Source: CAD feature listing. Evaluate the final solid. Frame: model axes, mm. Give positions to 0.01 mm unless a question says otherwise; leave off trailing zeros. Write each loop counter-clockwise with the first axis right and the second up, starting at its lowest first coordinate (ties: lowest second). Pieces come first, ordered by that corner, then holes. Notation, with made-up numbers: M 42.25,3 L 70.25,3 A22 cw 70.25,36 Z; hole C 70.25,51.5 d10. An arc over 180 degrees is marked long. Answer as a JSON object with one key per item and string values. Group by question number.
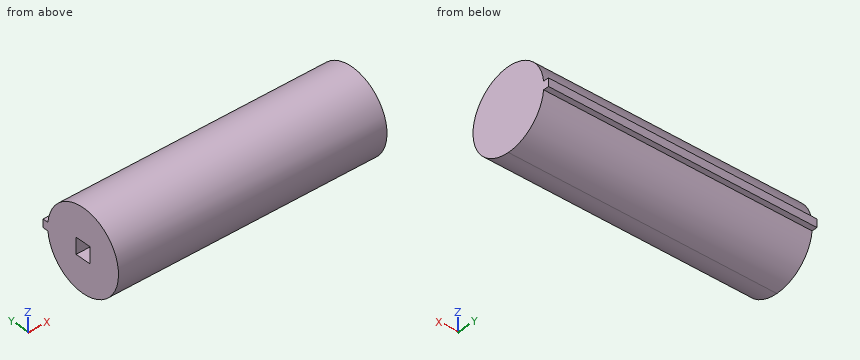
```python
from build123d import *

# Parameters (mm, degrees)
EXTRUDE_1_DEPTH     = 100
SKETCH_2_W          = 6
SKETCH_2_H          = 6
CUT_EXTRUDE_1_DEPTH = 15


with BuildPart() as part:
    # 草图1 → 凸台-拉伸1 (new body)
    with BuildSketch(Plane(origin=(0, 0, 0), x_dir=(0, 0, -1), z_dir=(1, 0, 0))):
        with BuildLine():
            Line((-1.5, 14.924811557), (-1.5, 0))
            Line((-1.5, 0), (1.5, 0))
            Line((1.5, 0), (1.5, 14.924811557))
            ThreePointArc((1.5, 14.924811557), (0, 15), (-1.5, 14.924811557))
        make_face()
        with BuildLine():
            Line((1.5, 0), (-1.5, 0))
            Line((-1.5, 0), (-1.5, 14.924811557))
            ThreePointArc((-1.5, 14.924811557), (-10.062305899, -11.124297731), (15, 0))
            ThreePointArc((15, 0), (11.124297731, 10.062305899), (1.5, 14.924811557))
            Line((1.5, 14.924811557), (1.5, 0))
        make_face()
        with BuildLine():
            Line((-1.5, 17), (-1.5, 14.924811557))
            ThreePointArc((-1.5, 14.924811557), (0, 15), (1.5, 14.924811557))
            Line((1.5, 14.924811557), (1.5, 17))
            Line((1.5, 17), (-1.5, 17))
        make_face()
    extrude(amount=EXTRUDE_1_DEPTH)

    # 草图2 → 切除-拉伸1 (cut)
    with BuildSketch(Plane.ZY):
        Rectangle(SKETCH_2_W, SKETCH_2_H)
    extrude(amount=-CUT_EXTRUDE_1_DEPTH, mode=Mode.SUBTRACT)


solid = part.part
```
(1) Section C-C, the plane y = 5. Return loops of the section in (x, z).
(2) Section A-A, the plane x = 70. Return loops of the section in (y, z), plus the area to 3 significant figures.
(3) Section B-B, the plane z = 0. Return loops of the section in (x, y).
(4) Contact query for flat-ended pins moving along their axis: pin 1 Ø1 at (x, y) = (60.5, 15.5) entering from +Z; pin 2 Ø6 at (x, z) = (22.5, -11.5) entering from +Y; pin 3 Ø10 at (x, y) = (12.5, 3.5) entering from -Z; pin 4 Ø8 at (x, z) = (45.5, -7.5) entering from +Y. Output: stop coordinate, or through.
(5) Section D-D, the plane z = 12. Return loops of the section in (x, y), plus the area to 3 significant figures.
(6) Ray query, L1, parallel to Z at x = 86, y = 15; L2, parallel to Z at x = 76.5, y = -6; L3, parallel to Y at x = 47.5, z = 11. Return the intervals inside material, ascending. Write a range as [from, to].
Reported:
{
 "1": {"outline": "M 0,-14.14 L 100,-14.14 L 100,14.14 L 0,14.14 Z"},
 "2": {"outline": "M 14.92,-1.5 L 17,-1.5 L 17,1.5 L 14.92,1.5 A15 ccw long Z", "area": "713 mm2"},
 "3": {"outline": "M 0,-15 L 100,-15 L 100,17 L 0,17 L 0,3 L 15,3 L 15,-3 L 0,-3 Z"},
 "4": {"pin 1": "stops at z = 1.5", "pin 2": "stops at y = 12.36", "pin 3": "stops at z = -15", "pin 4": "stops at y = 14.59"},
 "5": {"outline": "M 0,-9 L 100,-9 L 100,9 L 0,9 Z", "area": "1,800 mm2"},
 "6": {"L1": "z = [-1.5, 1.5]", "L2": "z = [-13.75, 13.75]", "L3": "y = [-10.2, 10.2]"}
}
